The listing builds one solid part. Answer for the finished solid, in the listing's coordinates (mm). Face numbers are marked on the shaded views. Give positions to 0.01 mm unless a question says otherwise; leave off trailing zeros. Order: outer loops, then holes, each group sorted by start corner. A loop starts at its lowest first (then second) coordinate and runs counter-clockwise, first axis right, second up. Notation, with made-up numbers: (-9, 38.25) - (14, 38.25) arc R22 ccw to (14, 69.25) - close; hole circle Ø3 at (-12, 71.25). An arc over 180 degrees is marked (long way). Answer as a JSON object with one key per item and string values. Group by question number.
Q1. A cutting plane is placed at A-A, the plane x = -123. Give the vertices of the cut face in (y, z), and give its area (3 significant figures).
Q2. The mould has two halves that part along X. Classify the marked faces 1 and 2: released by +X, released by -X, zero draft, split by the parting line, or undercut.
Q3. A cutting plane is placed at D-D, the plane x = -94. Give the vertices of the cut face in (y, z).
Q4. A cutting plane is placed at C-C, the plane x = -27. Give the vertices of the cut face in (y, z), and give its area (3 significant figures).
Q5. A cutting plane is placed at B-B, the plane z = 4. Count the separate pieces of the cut face and the enclosed holes in it, and give its area (3 significant figures).
Q6. Given pin 1 (1.2 mm diameter, centred on y = 3, z = 2.5, fed in from -X); pin 2 (3 mm diameter, centred on y = 25.5, z = 0.5, fed in from -X); pin 3 (1.2 mm diameter, centred on x = -122.5, z = 2, fed in from -Y); pin 4 (4 mm diameter, centred on x = -84.5, y = 6, fed in from -Z), each flat-ended and moving along its own axis, determine where each tip first touches the part or whether it passes through.
Q7. Consider line 1 (Y direction, x = -5, z = -0.75); line 2 (Y direction, x = -84, z = 3.5); line 3 (X direction, y = 18.5, z = 5.5). Determine where each line is inside the solid, lowest interval first.
Autodesk Inventor part; units mm, degrees
ref_plane "YZ Plane" through (0, 0, 0) normal (1, 0, 0) x (0, 1, 0)
ref_plane "XZ Plane" through (0, 0, 0) normal (0, 1, 0) x (-1, 0, 0)
ref_plane "XY Plane" through (0, 0, 0) normal (0, 0, 1) x (1, 0, 0)
sketch "Sketch1" plane through (0, 0, 0) normal (0, 0, 1) x (1, 0, 0)
  line L0 (-64, 31) -> (-73, 31)
  line L1 (-76, 28) -> (-76, 25)
  line L2 (-85, 16) -> (-76, 25)
  line L3 (-76, 28) -> (-73, 31)
  line L4 (-64, 31) -> (-55, 31)
  line L5 (-52, 28) -> (-52, 25)
  line L6 (-43, 16) -> (-52, 25)
  line L7 (-52, 28) -> (-55, 31)
  line L8 (-43, 16) -> (0, 16)
  line L9 (-77, 0) -> (-77, 5)
  line L10 (-77, 5) -> (-51, 5)
  line L11 (-51, 5) -> (-51, 0)
  line L12 (-106, 16) -> (-106, 7)
  line L13 (-106, 7) -> (-96, 7)
  line L14 (-96, 7) -> (-96, 16)
  line L15 (-128, 16) -> (-106, 16)
  line L16 (-96, 16) -> (-85, 16)
  line L17 (-120, 0) -> (-120, 7)
  line L18 (-120, 7) -> (-128, 7)
  line L19 (-120, 0) -> (-77, 0)
  line L20 (-128, 16) -> (-128, 7)
  line L21 (-8, 0) -> (-8, 7)
  line L22 (-8, 7) -> (0, 7)
  line L23 (-51, 0) -> (-8, 0)
  line L24 (0, 7) -> (0, 16)
  point P0 (0, 0)
  dimension "d0" = 128
  dimension "d6" = 3
  dimension "d67" = 5
  dimension "d71" = 22
  dimension "d74" = 9
  dimension "d75" = 10
  dimension "d93" = 7
  dimension "d94" = 8
  dimension "d95" = 7
extrude "Extrusion1" add sketch "Sketch1" against normal blind 2
sketch "Sketch2" plane through (0, 0, 0) normal (0, 0, 1) x (1, 0, 0)
  line L0 (-119, 2) -> (-113, 2)
  line L1 (-113, 2) -> (-113, 12)
  line L2 (-113, 12) -> (-119, 12)
  line L3 (-119, 12) -> (-119, 2)
  line L4 (-121, 10) -> (-125, 10)
  line L5 (-125, 10) -> (-125, 14)
  line L6 (-125, 14) -> (-121, 14)
  line L7 (-121, 14) -> (-121, 10)
  line L8 (-88, 2) -> (-82, 2)
  line L9 (-82, 2) -> (-82, 12)
  line L10 (-82, 12) -> (-88, 12)
  line L11 (-88, 12) -> (-88, 2)
  line L12 (-90, 0) -> (-80, 0)
  line L13 (-80, 0) -> (-80, 14)
  line L14 (-80, 14) -> (-90, 14)
  line L15 (-90, 14) -> (-90, 0)
  line L16 (-99, 1) -> (-103, 1)
  line L17 (-103, 1) -> (-103, 5)
  line L18 (-103, 5) -> (-99, 5)
  line L19 (-99, 5) -> (-99, 1)
  line L20 (-61, 26) -> (-67, 26)
  line L21 (-67, 26) -> (-67, 16)
  line L22 (-67, 16) -> (-61, 16)
  line L23 (-61, 16) -> (-61, 26)
  line L24 (-59, 14) -> (-69, 14)
  line L25 (-69, 14) -> (-69, 28)
  line L26 (-69, 28) -> (-59, 28)
  line L27 (-59, 28) -> (-59, 14)
  line L28 (-9, 2) -> (-15, 2)
  line L29 (-15, 2) -> (-15, 12)
  line L30 (-15, 12) -> (-9, 12)
  line L31 (-9, 12) -> (-9, 2)
  line L32 (-7, 10) -> (-3, 10)
  line L33 (-3, 10) -> (-3, 14)
  line L34 (-3, 14) -> (-7, 14)
  line L35 (-7, 14) -> (-7, 10)
  line L36 (-40, 2) -> (-46, 2)
  line L37 (-46, 2) -> (-46, 12)
  line L38 (-46, 12) -> (-40, 12)
  line L39 (-40, 12) -> (-40, 2)
  line L40 (-38, 0) -> (-48, 0)
  line L41 (-48, 0) -> (-48, 14)
  line L42 (-48, 14) -> (-38, 14)
  line L43 (-38, 14) -> (-38, 0)
  line L44 (-29, 1) -> (-25, 1)
  line L45 (-25, 1) -> (-25, 5)
  line L46 (-25, 5) -> (-29, 5)
  line L47 (-29, 5) -> (-29, 1)
  line L48 (-112, 13) -> (-120, 13)
  line L49 (-8, 13) -> (-16, 13)
  line L50 (-120, 13) -> (-120, 0)
  line L51 (-112, 13) -> (-112, 0)
  line L52 (-16, 13) -> (-16, 0)
  line L53 (-8, 13) -> (-8, 0)
  circle A0 centre (-123, 12) radius 1.25
  circle A1 centre (-101, 3) radius 1.25
  circle A2 centre (-27, 3) radius 1.25
  circle A3 centre (-5, 12) radius 1.25
  line L54 (-120, 0) -> (-112, 0)
  line L55 (-16, 0) -> (-8, 0)
  dimension "d12" = 6
  dimension "d13" = 10
  dimension "d21" = 6
  dimension "d22" = 10
  dimension "d23" = 2
  dimension "d29" = 6
  dimension "d30" = 10
  dimension "d31" = 2
  dimension "d48" = 1
  dimension "d49" = 2.5
  dimension "d50" = 2.5
  dimension "d51" = 2.5
  dimension "d52" = 2.5
  dimension "d69" = 13
sketch "Sketch10" plane through (0, 0, 0) normal (0, 0, 1) x (1, 0, 0)
  line L0 (-119, 2) -> (-113, 2)
  line L1 (-113, 2) -> (-113, 12)
  line L2 (-113, 12) -> (-119, 12)
  line L3 (-119, 12) -> (-119, 2)
  line L4 (-121, 10) -> (-125, 10)
  line L5 (-125, 10) -> (-125, 14)
  line L6 (-125, 14) -> (-121, 14)
  line L7 (-121, 14) -> (-121, 10)
  line L8 (-88, 2) -> (-82, 2)
  line L9 (-82, 2) -> (-82, 12)
  line L10 (-82, 12) -> (-88, 12)
  line L11 (-88, 12) -> (-88, 2)
  line L12 (-90, 0) -> (-80, 0)
  line L13 (-80, 0) -> (-80, 14)
  line L14 (-80, 14) -> (-90, 14)
  line L15 (-90, 14) -> (-90, 0)
  line L16 (-99, 1) -> (-103, 1)
  line L17 (-103, 1) -> (-103, 5)
  line L18 (-103, 5) -> (-99, 5)
  line L19 (-99, 5) -> (-99, 1)
  line L20 (-61, 26) -> (-67, 26)
  line L21 (-67, 26) -> (-67, 16)
  line L22 (-67, 16) -> (-61, 16)
  line L23 (-61, 16) -> (-61, 26)
  line L24 (-59, 14) -> (-69, 14)
  line L25 (-69, 14) -> (-69, 28)
  line L26 (-69, 28) -> (-59, 28)
  line L27 (-59, 28) -> (-59, 14)
  line L28 (-25, 1) -> (-25, 5)
  line L29 (-9, 2) -> (-15, 2)
  line L30 (-15, 2) -> (-15, 12)
  line L31 (-15, 12) -> (-9, 12)
  line L32 (-9, 12) -> (-9, 2)
  line L33 (-7, 14) -> (-7, 10)
  line L34 (-7, 10) -> (-3, 10)
  line L35 (-3, 10) -> (-3, 14)
  line L36 (-3, 14) -> (-7, 14)
  line L37 (-29, 1) -> (-25, 1)
  line L38 (-25, 5) -> (-29, 5)
  line L39 (-29, 5) -> (-29, 1)
  line L40 (-38, 14) -> (-38, 0)
  line L41 (-40, 12) -> (-40, 2)
  line L42 (-40, 2) -> (-46, 2)
  line L43 (-46, 12) -> (-40, 12)
  line L44 (-46, 2) -> (-46, 12)
  line L45 (-48, 14) -> (-38, 14)
  line L46 (-48, 0) -> (-48, 14)
  line L47 (-38, 0) -> (-48, 0)
  line L48 (-112, 13) -> (-120, 13)
  line L49 (-8, 13) -> (-16, 13)
  circle A0 centre (-123, 12) radius 1.25
  circle A1 centre (-101, 3) radius 1.25
  circle A2 centre (-27, 3) radius 1.25
  circle A3 centre (-5, 12) radius 1.25
  line L50 (-120, 13) -> (-120, 0)
  line L51 (-112, 13) -> (-112, 0)
  line L52 (-112, 0) -> (-120, 0)
  line L53 (-16, 13) -> (-16, 0)
  line L54 (-16, 0) -> (-8, 0)
  line L55 (-8, 13) -> (-8, 0)
  point P0 (-100.5385, 17.107)
  point P1 (-110.5385, 3.107)
  point P2 (-100.5385, 3.107)
  point P3 (-141.5385, 3.107)
  point P4 (-131.5385, 3.107)
  point P5 (-183.5385, 3.107)
  point P6 (-173.5385, 3.107)
  point P7 (-214.5385, 3.107)
  point P8 (-204.5385, 3.107)
  point P9 (-214.5385, 17.107)
  point P10 (0, 16)
  point P11 (0, 0)
  dimension "d53" = 6
  dimension "d54" = 10
  dimension "d55" = 6
  dimension "d56" = 10
  dimension "d57" = 2
  dimension "d58" = 6
  dimension "d59" = 10
  dimension "d60" = 2
  dimension "d61" = 1
  dimension "d62" = 2.5
  dimension "d63" = 2.5
  dimension "d64" = 2.5
  dimension "d65" = 2.5
extrude "Extrusion2" cut sketch "Sketch2" against normal blind 2 contours L3 L2 L1 L0 | L11 L10 L9 L8 | L23 L22 L21 L20 | L28 L29 L30 L31 | L36 L37 L38 L39 | A0 | A1 | A2 | A3
extrude "Extrusion7" add sketch "Sketch10" along normal blind 6
properties part number "Infravermelhos_revisto_2"
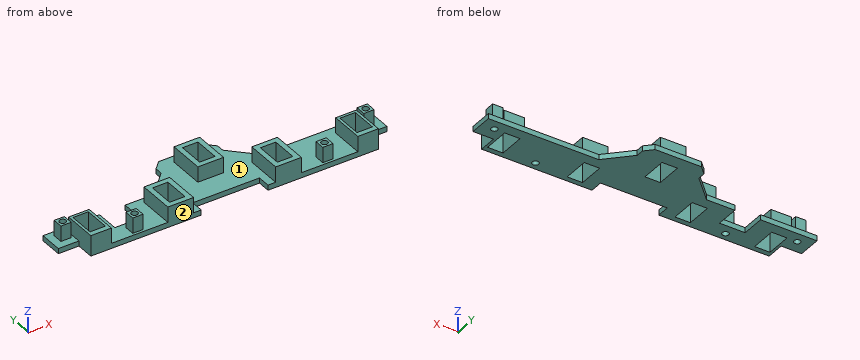
Reply:
{
 "1": {"outline": "(7, -2) - (10.75, -2) - (10.75, 6) - (10, 6) - (10, 0) - (7, 0) - close; (13.25, -2) - (16, -2) - (16, 0) - (14, 0) - (14, 6) - (13.25, 6) - close", "area": "22.0 mm^2"},
 "2": {"face 1": "undercut", "face 2": "zero draft"},
 "3": {"outline": "(0, -2) - (16, -2) - (16, 0) - (0, 0) - close"},
 "4": {"outline": "(0, -2) - (1.75, -2) - (1.75, 6) - (1, 6) - (1, 0) - (0, 0) - close; (4.25, -2) - (16, -2) - (16, 0) - (5, 0) - (5, 6) - (4.25, 6) - close", "area": "36.0 mm^2"},
 "5": {"separate pieces": "9", "enclosed holes": "9", "area": "372 mm^2"},
 "6": {"pin 1": "stops at x = -120", "pin 2": "stops at x = -76.91", "pin 3": "stops at y = 10", "pin 4": "passes through"},
 "7": {"line 1": "y = 7 to 10.75, 13.25 to 16", "line 2": "y = 0 to 2, 12 to 14", "line 3": "x = -69 to -67, -61 to -59"}
}
